The listing builds one solid part. Answer for the finished solid, in the listing's coordinates (mm). Face numbers are marked on the shaded views. A direction names the side the tool comes from. Coordinates: 2 decimals unless noted, no trailing zeros. Write each loop counter-clockwise with the first axis right and the second up, starting at its lowest first coordinate (ties: lowest second). Pieces come first, ordered by that corner, then holes.
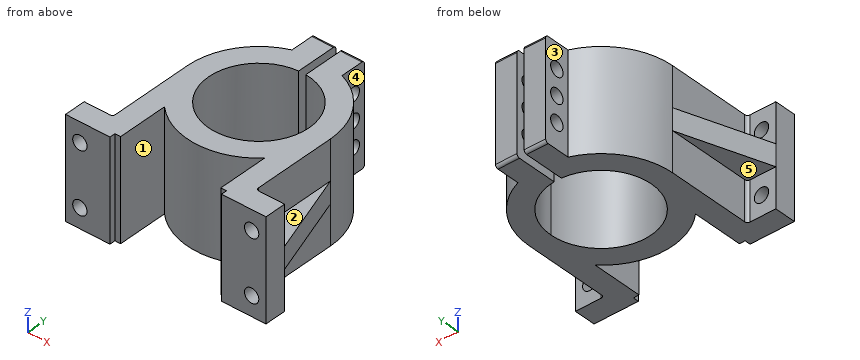
from build123d import *

# Parameters (mm, degrees)
SKETCH1_R                = 20
SKETCH1_R_2              = 14
BOSS_EXTRUDE1_DEPTH      = 14
BOSS_EXTRUDE2_DEPTH      = 28
SKETCH3_W                = 1.6
SKETCH3_H                = 1.6
CUT_EXTRUDE1_DEPTH       = 50.678969393
FILLET1_R                = 0.8
BOSS_EXTRUDE3_DEPTH      = 14
BOSS_EXTRUDE3_DEPTH_BACK = 14
SKETCH5_W                = 2
SKETCH5_H                = 28
CUT_EXTRUDE2_DEPTH       = 25
SKETCH6_R                = 2
CUT_EXTRUDE3_DEPTH       = 49.176757882
FILLET2_R                = 0.8
RIB1_REACH               = 45.359
SKETCH7_WALL_W           = 114.016154836
SKETCH7_WALL_H           = 6
SKETCH8_R                = 2
CUT_EXTRUDE4_DEPTH       = 59.936437162
SKETCH9_W                = 2
SKETCH9_H                = 14
CUT_EXTRUDE5_DEPTH       = 31


with BuildPart() as part:
    # Sketch1 → Boss-Extrude1 (new, symmetric)
    with BuildSketch(Plane.XY):
        Circle(SKETCH1_R)
        Circle(SKETCH1_R_2, mode=Mode.SUBTRACT)
    extrude(amount=BOSS_EXTRUDE1_DEPTH, both=True)

    # Sketch2 → Boss-Extrude2 (add)
    with BuildSketch(Plane.XY.offset(14)):
        with BuildLine():
            Line((-20, 0), (-20, -24))
            Line((-20, -24), (-28, -24))
            Line((-28, -24), (-28, -30))
            Line((-28, -30), (-14, -30))
            Line((-14, -30), (-14, -14.282856857))
            ThreePointArc((-14, -14.282856857), (-18.439088915, -7.745966692), (-20, 0))
        make_face()
        with BuildLine():
            Line((14, -30), (14, -14.282856857))
            ThreePointArc((14, -14.282856857), (18.439088915, -7.745966692), (20, 0))
            Line((20, 0), (20, -24))
            Line((20, -24), (28, -24))
            Line((28, -24), (28, -30))
            Line((28, -30), (14, -30))
        make_face()
    extrude(amount=-BOSS_EXTRUDE2_DEPTH)

    # Sketch3 → Cut-Extrude1 (cut, through all)
    with BuildSketch(Plane.XY.offset(14)):
        with Locations((-14.8, -29.2)):
            Rectangle(SKETCH3_W, SKETCH3_H)
        with Locations((14.8, -29.2)):
            Rectangle(SKETCH3_W, SKETCH3_H)
    extrude(amount=-CUT_EXTRUDE1_DEPTH, mode=Mode.SUBTRACT)

    # Fillet1
    fillet1_edges = [part.edges().sort_by_distance(p)[0] for p in [
        (-20, -24, 0),
        (20, -24, 0),
    ]]
    fillet(fillet1_edges, radius=FILLET1_R)

    # Sketch4 → Boss-Extrude3 (add, two sides: drawn at the far end of the back side and taken through both)
    with BuildSketch(Plane.XY.offset(-BOSS_EXTRUDE3_DEPTH_BACK)):
        with BuildLine():
            Line((-7, 18.734993995), (-7, 25.934993995))
            Line((-7, 25.934993995), (7, 25.934993995))
            Line((7, 25.934993995), (7, 18.734993995))
            ThreePointArc((7, 18.734993995), (0, 20), (-7, 18.734993995))
        make_face()
    extrude(amount=BOSS_EXTRUDE3_DEPTH + BOSS_EXTRUDE3_DEPTH_BACK)

    # Sketch5 → Cut-Extrude2 (cut)
    with BuildSketch(Plane(origin=(0, 25.934993995, 0), x_dir=(1, 0, 0), z_dir=(0, 1, 0))):
        with Locations((0, -14)):
            Rectangle(SKETCH5_W, SKETCH5_H)
    extrude(amount=-CUT_EXTRUDE2_DEPTH, mode=Mode.SUBTRACT)

    # Sketch6 → Cut-Extrude3 (cut, through all)
    with BuildSketch(Plane(origin=(7, 0, 0), x_dir=(0, 0, -1), z_dir=(1, 0, 0))):
        with Locations((0, 22.334993995)):
            Circle(SKETCH6_R)
        with Locations((-7, 22.334993995)):
            Circle(SKETCH6_R)
        with Locations((7, 22.334993995)):
            Circle(SKETCH6_R)
    extrude(amount=-CUT_EXTRUDE3_DEPTH, mode=Mode.SUBTRACT)

    # Fillet2
    fillet2_edges = [part.edges().sort_by_distance(p)[0] for p in [
        (-4, 25.934993995, 14),
        (0, 25.934993995, -14),
        (4, 25.934993995, 14),
    ]]
    fillet(fillet2_edges, radius=FILLET2_R)

    # Sketch7 wall → Rib1 (add, up to next)
    with BuildSketch(Plane(origin=(24, -12, 0), x_dir=(0.316227766017, -0.948683298051, 0), z_dir=(0.948683298051, 0.316227766017, 0)), mode=Mode.PRIVATE) as rib1_sk1:
        Rectangle(SKETCH7_WALL_W, SKETCH7_WALL_H)
    rib1_tool1 = extrude(rib1_sk1.sketch, amount=-RIB1_REACH, mode=Mode.PRIVATE) - part.part
    rib1 = rib1_tool1.solids().sort_by_distance((24, -12, 0))[0]
    add(rib1)

    # Sketch8 → Cut-Extrude4 (cut, through all)
    with BuildSketch(Plane(origin=(0, -24, 0), x_dir=(1, 0, 0), z_dir=(0, 1, 0))):
        with Locations(Location((24, 8.5, 0), (0, 0, 270))):
            Circle(SKETCH8_R)
        with Locations(Location((24, -8.5, 0), (0, 0, 270))):
            Circle(SKETCH8_R)
    cut_extrude4 = extrude(amount=-CUT_EXTRUDE4_DEPTH, mode=Mode.SUBTRACT)

    # Mirror1: Rib1, Cut-Extrude4 across plane
    add(rib1.mirror(Plane(origin=(0, 0, 0), x_dir=(0, 0, 1), z_dir=(1, 0, 0))))
    add(cut_extrude4.mirror(Plane(origin=(0, 0, 0), x_dir=(0, 0, 1), z_dir=(1, 0, 0))), mode=Mode.SUBTRACT)

    # Sketch9 → Cut-Extrude5 (cut)
    with BuildSketch(Plane(origin=(0, 25.934993995, 0), x_dir=(1, 0, 0), z_dir=(0, 1, 0))):
        with Locations((0, 7)):
            Rectangle(SKETCH9_W, SKETCH9_H)
    extrude(amount=-CUT_EXTRUDE5_DEPTH, mode=Mode.SUBTRACT)


solid = part.part
1. Section A-A on z = 0 is taken. State how many separate pieces and enclosed holes the cut face has, then the cut area to 3 significant figures.
Results found:
separate pieces: 3
enclosed holes: 0
area: 1,180 mm2
2. Section C-C on y = -13 is taken. Give the vertices of the cut face in (x, z), then the cut area to 3 significant figures.
Results found:
outline: (-24.33, -3) - (-20, -3) - (-20, -14) - (-5.2, -14) - (-5.2, 14) - (-20, 14) - (-20, 3) - (-24.33, 3) - close; (5.2, -14) - (20, -14) - (20, -3) - (24.33, -3) - (24.33, 3) - (20, 3) - (20, 14) - (5.2, 14) - close
area: 881 mm2
3. Section B-B on x = 24 is taken. Give the vertices of the cut face in (y, z), then the cut area to 3 significant figures.
Results found:
outline: (-30, -14) - (-24, -14) - (-24, -10.5) - (-30, -10.5) - close; (-30, -6.5) - (-24, -6.5) - (-24, -3) - (-12, -3) - (-12, 3) - (-24, 3) - (-24, 6.5) - (-30, 6.5) - close; (-30, 10.5) - (-24, 10.5) - (-24, 14) - (-30, 14) - close
area: 192 mm2
4. Flat-ended cylindrical pins translate along their axes: P1, Ø1.5, axis at x = 11.5, z = -1, coming from the -Y side; P2, Ø5, axis at y = 0.5, z = 1, coming from the +X side; P3, Ø3.5, axis at y = -9.5, z = -10, coming from the +X side. Find the tip coordinate at first contact, or state that the pin passes through.
Results found:
P1: stops at y = -16.87
P2: stops at x = 20.67
P3: stops at x = 20
5. A tool of negligible diameter and unlimited length cuts with its end or side. For the marked faces 1, 2, 3, 4 and 5, from which of +Z, -Z, +X, -X, +Y, -Y can it reach the whole face along a straight path? Write none if from no direction.
Results found:
face 1: +Z, -Z, -Y
face 2: +Z, +X, +Y
face 3: +Z, -Z, -X, +Y
face 4: +Z, -Z, +X, +Y
face 5: -Z, -X, +Y
6. Find the intervals of material crossed by L1, parallel to Z at x = -24, y = -26.5; L2, parallel to X at y = -18, z = 6.25; L3, parallel to Y at x = -3.1, z = 7 (3 decimals), in increasing order.
Results found:
L1: z = -14 to -10.5, -6.5 to 6.5, 10.5 to 14
L2: x = -20 to -14, -8.72 to 8.72, 14 to 20
L3: y = -19.758 to -13.652, 13.652 to 20.335, 24.335 to 25.935
7. Section D-D on x = -9.5 is taken. Give the vertices of the cut face in (y, z), then the cut area to 3 significant figures.
Results found:
outline: (-17.6, -14) - (-10.28, -14) - (-10.28, 14) - (-17.6, 14) - close; (10.28, -14) - (17.6, -14) - (17.6, 14) - (10.28, 14) - close
area: 410 mm2
